Input: part model. Units: mm. Frame: model coordinates. Give positions to 0.01 mm unless a question says otherwise; leave off trailing zeros. Loops run counter-clockwise (first coordinate to the right, second up) from the corner with the lowest first, then second, coordinate; pieces in that order, holes last. Notation, with made-up numbers: (36.5, 66) -> (92.5, 66) arc R11 ccw to (92.5, 85) -> close; hole circle Ø8 at (9.5, 57). An arc over 180 degrees is marked (long way). One line per question, with ' | ' between items.
Autodesk Inventor part; units mm, degrees
ref_plane "a_XY" through (0, 0, 0) normal (1, 0, 0) x (0, 0, -1)
ref_plane "a_YZ" through (0, 0, 0) normal (0, 0, -1) x (0, 1, 0)
ref_plane "a_ZX" through (0, 0, 0) normal (0, 1, 0) x (1, 0, 0)
sketch "Sketch_1" plane through (0, 0, 0) normal (0, 0, 1) x (1, 0, 0)
  line L0 (-3, 0) -> (3, 0)
  line L1 (0, -6.2) -> (0, -7.8)
  line L2 (0, -7.8) -> (0.2, -8)
  line L3 (0.2, -8) -> (0.8, -8)
  line L4 (0.8, -8) -> (1, -7.8)
  line L5 (1, -7.8) -> (1, -6.2)
  line L6 (1, -6.2) -> (0.8, -6)
  line L7 (0.8, -6) -> (0.2, -6)
  line L8 (0.2, -6) -> (0, -6.2)
revolve "Revolution1" add sketch "Sketch_1" angle 360 about axis through (-3, 0, 0) along (-1, 0, 0)
ref_plane "a_XY" through (0, 0, 0) normal (1, 0, 0) x (0, 0, -1)
ref_plane "a_YZ" through (0, 0, 0) normal (0, 0, -1) x (0, 1, 0)
ref_plane "a_ZX" through (0, 0, 0) normal (0, 1, 0) x (1, 0, 0)
properties part number "WSSS16-12-1"
1. Section query C-C (x = 0.5). Output: boundary loops of the cut face in (y, z).
Determined:
outline: circle Ø16 at (0, 0); hole circle Ø12 at (0, 0)
2. Ray query, line 1 along Z through (x, y) = (0.55, 0); line 2 along Z through (x, y) = (0.75, -5.5); line 3 along Y through (x, z) = (0.15, -0.5). Return the intervals inside material, ascending. Write a range as from..to.
Determined:
line 1: z = -8..-6, 6..8 | line 2: z = -5.81..-2.4, 2.4..5.81 | line 3: y = -7.93..-6.03, 6.03..7.93
3. Pull-direction query (Z, two-part tool) for faces 1 (the cylindrical face through (0.5, 1.73, 7.81)), 2 (the cylindrical face through (0.496, 5.994, 0.264)), 3 (the flat face through (1, 3, -6)); classes: pulls with the +Z half, pulls with the -Z half, needs draft (parallel to the pull), parting line crosses it, or undercut.
Determined:
face 1: parting line crosses it | face 2: undercut | face 3: needs draft
4. Pin query (flat end, axial travel): P1, Ø3, axis at y = 1.5, z = -2, coming from the -X side. Return the tip coordinate at first contact, or that it passes through.
Determined:
P1: passes through
5. Section query A-A (z = 0). Output: boundary loops of the cut face in (x, y), then the cut area to 3 significant figures.
Determined:
outline: (0, -7.8) -> (0.2, -8) -> (0.8, -8) -> (1, -7.8) -> (1, -6.2) -> (0.8, -6) -> (0.2, -6) -> (0, -6.2) -> close; (0, 6.2) -> (0.2, 6) -> (0.8, 6) -> (1, 6.2) -> (1, 7.8) -> (0.8, 8) -> (0.2, 8) -> (0, 7.8) -> close | area: 3.84 mm2
